Part model, mm, in its own coordinate system. Coordinates: 2 decimals unless noted, no trailing zeros. Order: outer loops, then holes, each group sorted by start corner. A loop starts at its lowest first (then second) coordinate and runs counter-clockwise, first axis right, second up.
from build123d import *

# Parameters (mm, degrees)
BOSS_EXTRUDE1_DEPTH = 2.38125
SKETCH3_OUTSIDE_W   = 129.43
SKETCH3_OUTSIDE_H   = 120.054
CUT_EXTRUDE1_DEPTH  = 2.38125


with BuildPart() as part:
    # Sketch2 → Boss-Extrude1 (new, symmetric)
    with BuildSketch(Plane(origin=(0, 0, 0), x_dir=(1, 0, 0), z_dir=(0, 1, 0))):
        with BuildLine():
            Line((-29.2030912, -40.788560766), (29.2030912, -40.788560766))
            ThreePointArc((29.2030912, -40.788560766), (0, 50.165), (-29.2030912, -40.788560766))
        make_face()
    extrude(amount=BOSS_EXTRUDE1_DEPTH, both=True)

    # Sketch3 outside → Cut-Extrude1 (cut)
    with BuildSketch(Plane.XZ.offset(2.38125)):
        with Locations((0, -4.688)):
            Rectangle(SKETCH3_OUTSIDE_W, SKETCH3_OUTSIDE_H)
        with BuildLine():
            Line((-28.428247287, 38.407310766), (28.428247287, 38.407310766))
            ThreePointArc((28.428247287, 38.407310766), (0, -47.78375), (-28.428247287, 38.407310766))
        make_face(mode=Mode.SUBTRACT)
    extrude(amount=-CUT_EXTRUDE1_DEPTH, mode=Mode.SUBTRACT)


solid = part.part
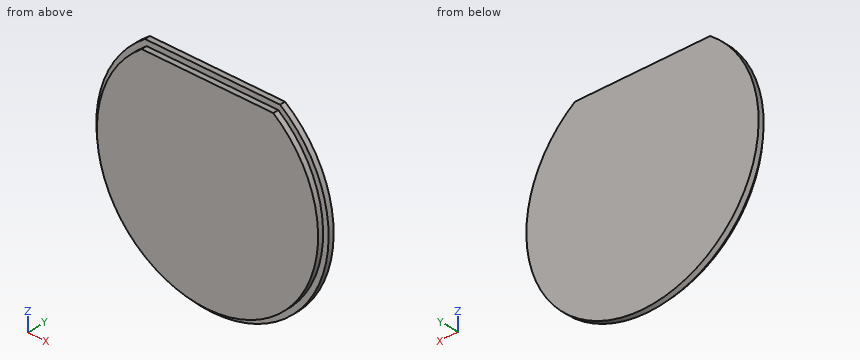
Q1. Cut at C-C on y = 1.25. Write the cut outline in (x, z) (3 decimals), and give its area (3 significant figures).
Results list:
outline: (-29.203, 40.789) arc R50.165 ccw (long way) to (29.203, 40.789) - close
area: 7,530 mm2
Q2. Cut at B-B on x = 0. Write the cut outline in (y, z) (3 decimals), and give its area (3 significant figures).
Results list:
outline: (-2.381, -47.784) - (0, -47.784) - (0, -50.165) - (2.381, -50.165) - (2.381, 40.789) - (0, 40.789) - (0, 38.407) - (-2.381, 38.407) - close
area: 422 mm2
Q3. Cut at A-A on z = 0. Write the cut outline in (x, y) (3 decimals), and give its area (3 significant figures).
Results list:
outline: (-50.165, 0) - (-47.784, 0) - (-47.784, -2.381) - (47.784, -2.381) - (47.784, 0) - (50.165, 0) - (50.165, 2.381) - (-50.165, 2.381) - close
area: 466 mm2
Q4. Wall check: line 1 along Y through (x, z) = (-32, -38.5); line 2 along Z through (x, y) = (1.5, 1.55); line 3 along X through (y, z) = (-1.3, 4.5). Give the ranges that are in metal, low to high.
Results list:
line 1: y = 0 to 2.38
line 2: z = -50.14 to 40.79
line 3: x = -47.57 to 47.57
Q5. Pin check, flat tips, straight feed: pin 1 Ø2 at (x, y) = (-33.5, -1.5) entering from -Z; pin 2 Ø2 at (x, y) = (14, -1.5) entering from -Z; pin 3 Ø2 at (y, z) = (-1.5, 20.5) entering from -X. Stop position of each tip, or through.
Results list:
pin 1: stops at z = -35.03
pin 2: stops at z = -45.98
pin 3: stops at x = -43.62
